Part model, mm, in its own coordinate system. A direction names the side the tool comes from. Give positions to 0.01 mm unless a question says otherwise; leave off trailing zeros. Order: outer loops, then holes, each group sorted by start corner. A loop starts at its lowest first (then second) coordinate and runs counter-clockwise, first axis right, second up. Notation, with made-up numbers: M 28.25,11 L 67.25,11 A23 ccw 67.25,19 Z; hole C -1,34 d4. An arc over 180 degrees is marked long. Return JSON: item names as keys, results as strings.
from build123d import *

# Parameters (mm, degrees)
SKETCH1_W           = 100
SKETCH1_H           = 100
SKETCH1_W_2         = 88
SKETCH1_H_2         = 88
BOSS_EXTRUDE1_DEPTH = 30
SKETCH2_R           = 7.5
CUT_EXTRUDE1_DEPTH  = 145.568322948


with BuildPart() as part:
    # Sketch1 → Boss-Extrude1 (new body)
    with BuildSketch(Plane(origin=(0, 0, 0), x_dir=(1, 0, 0), z_dir=(0, 1, 0))):
        with Locations((50, 50)):
            Rectangle(SKETCH1_W, SKETCH1_H)
        with Locations((50, 50)):
            Rectangle(SKETCH1_W_2, SKETCH1_H_2, mode=Mode.SUBTRACT)
    extrude(amount=BOSS_EXTRUDE1_DEPTH)

    # Sketch2 → Cut-Extrude1 (cut, through all)
    with BuildSketch(Plane.XY):
        with Locations((50, 15)):
            Circle(SKETCH2_R)
    extrude(amount=-CUT_EXTRUDE1_DEPTH, mode=Mode.SUBTRACT)


solid = part.part
Q1. Band-saw the part on C-C (z = -84.5). Give the cut face in (x, y).
Established:
{"outline": "M 0,0 L 6,0 L 6,30 L 0,30 Z; M 94,0 L 100,0 L 100,30 L 94,30 Z"}
Q2. 3-axis set-ups, long thin cutter, end or side, ignore diameter. For faces 1 (the flat face through (0, 15, -49)), 2 (the flat face through (94, 15, -49)): which of +Z, -Z, +X, -X, +Y, -Y reach the whole face in a straight line?
Established:
{"face 1": "+Z, -Z, -X, +Y, -Y", "face 2": "+Y, -Y"}
Q3. Probe line 1 along Z through (x, y) = (9, 10.5); line 2 along X through (y, z) = (28, -8.5); line 3 along Y through (x, z) = (50, -96.4). List the from-to ranges inside material, lowest first.
Established:
{"line 1": "z = -100 to -94, -6 to 0", "line 2": "x = 0 to 6, 94 to 100", "line 3": "y = 0 to 7.5, 22.5 to 30"}
Q4. Band-saw the part on B-B (x = 89). Give the cut face in (y, z), then the cut area to 3 significant figures.
Established:
{"outline": "M 0,-100 L 30,-100 L 30,-94 L 0,-94 Z; M 0,-6 L 30,-6 L 30,0 L 0,0 Z", "area": "360 mm²"}
Q5. Pin check, flat tip, straight feed: pin 1 (5 mm diameter, centred on x = 31.5, z = -89.5, fed in from +Y). Stop position of the tip, or through.
Established:
{"pin 1": "passes through"}
Q6. Band-saw the part on A-A (y = 15). Give the cut face in (x, z).
Established:
{"outline": "M 0,-100 L 42.5,-100 L 42.5,-94 L 6,-94 L 6,-6 L 42.5,-6 L 42.5,0 L 0,0 Z; M 57.5,-100 L 100,-100 L 100,0 L 57.5,0 L 57.5,-6 L 94,-6 L 94,-94 L 57.5,-94 Z"}
Q7. Two-plate mould, pull along X, no slides. Class faces 3 (the cylindrical face through (57.154, 17.253, -96.958)), 4 (the flat face through (5, 30, -50)), 5 (the cylindrical face through (57.154, 17.253, -2.958)), 6 (the flat face through (100, 15, -49)): +X half, -X half, draft (parallel to the pull), parting line (faces both ways), or undercut.
Established:
{"face 3": "undercut", "face 4": "draft", "face 5": "undercut", "face 6": "+X half"}
Q8. Band-saw the part on D-D (y = 24.25). Give the cut face in (x, z).
Established:
{"outline": "M 0,-100 L 100,-100 L 100,0 L 0,0 Z; hole M 6,-94 L 94,-94 L 94,-6 L 6,-6 Z"}
